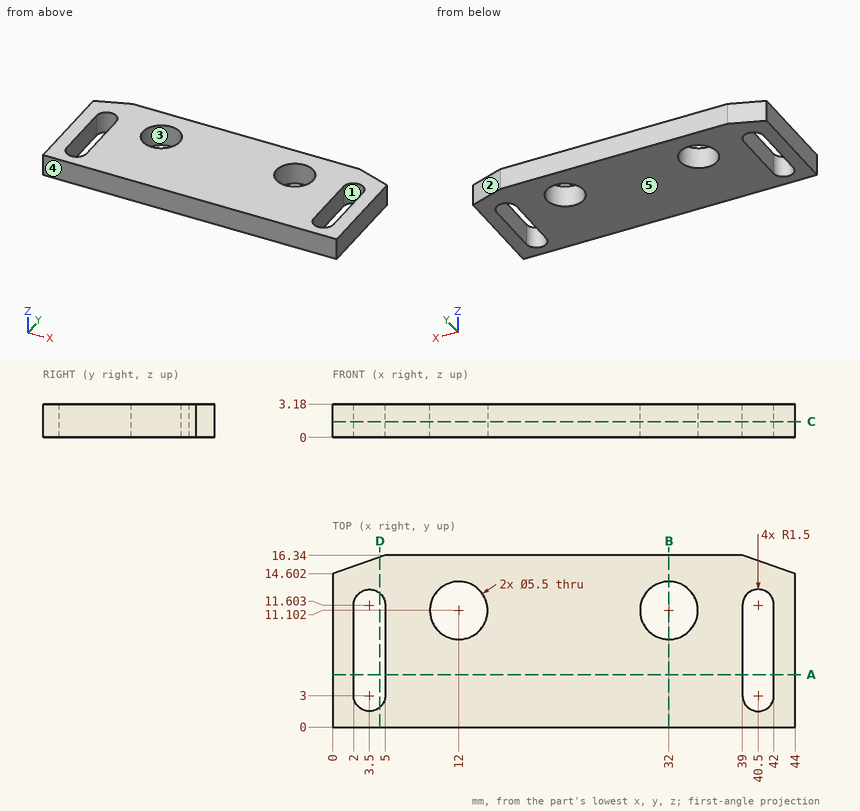
Source: three-view drawing plus pictorial views. Frame: mm from the lowest corner of the part. A direction names the side the tool comes from. Round coordinates to 2 decimals unless told otherwise and drop trailing zeros. Write each loop counter-clockwise with the first axis right and the second up, starting at its lowest first coordinate (ties: lowest second). Pieces come first, ordered by that corner, then holes. Notation, with made-up numbers: M 47,39 L 74,39 A9 ccw 74,49 Z; hole C 50,-33 d1. An arc over 180 degrees is marked long. Write each question's results on one line, items separated by ' | '.
Q1. Pin query (flat end, axial travel): P1, Ø6.5, axis at x = 32, y = 11.1, coming from the -Z side. Return the tip coordinate at first contact, or that it passes through.
Results:
P1: stops at z = 0
Q2. Section query C-C (z = 1.5). Return loops of the section in (x, y), and give its area (3 significant figures).
Results:
outline: M 0,0 L 44,0 L 44,14.6 L 39,16.34 L 5,16.34 L 0,14.6 Z; hole M 2,3 A1.5 ccw 5,3 L 5,11.6 A1.5 ccw 2,11.6 Z; hole C 12,11.1 d5.5; hole C 32,11.1 d5.5; hole M 39,3 A1.5 ccw 42,3 L 42,11.6 A1.5 ccw 39,11.6 Z | area: 597 mm^2
Q3. Section query B-B (x = 32). Return loops of the section in (y, z).
Results:
outline: M 0,0 L 8.35,0 L 8.35,3.18 L 0,3.18 Z; M 13.85,0 L 16.34,0 L 16.34,3.18 L 13.85,3.18 Z
Q4. Access query for the marked faces 1 and 2. Directions: +Z, -Z, +X, -X, +Y, -Y. A direction counts if a zero-diameter tool reaches every point of the face in a straight line with its end or side. Return the directions, or none.
Results:
face 1: +Z, -Z | face 2: +Z, -Z, +X, +Y
Q5. Section query D-D (x = 4.5). Return loops of the section in (y, z).
Results:
outline: M 0,0 L 1.88,0 L 1.88,3.18 L 0,3.18 Z; M 12.72,0 L 16.17,0 L 16.17,3.18 L 12.72,3.18 Z
Q6. Section query A-A (y = 5). Return loops of the section in (x, z).
Results:
outline: M 0,0 L 2,0 L 2,3.18 L 0,3.18 Z; M 5,0 L 39,0 L 39,3.18 L 5,3.18 Z; M 42,0 L 44,0 L 44,3.18 L 42,3.18 Z
Q7. Draft query along Y for the marked faces 3, 4 and 5. Return one class per face: released by +Y, released by -Y, zero draft, split by the parting line, or undercut.
Results:
face 3: undercut | face 4: released by -Y | face 5: zero draft
Q8. Line query: line 1 along X through (y, z) = (11, 0.45); line 2 along X through (y, z) = (6.5, 3.05); line 3 along X through (y, z) = (12.5, 2.1). Output: solid intervals per line, ascending.
Results:
line 1: x = 0 to 2, 5 to 9.25, 14.75 to 29.25, 34.75 to 39, 42 to 44 | line 2: x = 0 to 2, 5 to 39, 42 to 44 | line 3: x = 0 to 2.3, 4.7 to 9.63, 14.37 to 29.63, 34.37 to 39.3, 41.7 to 44
